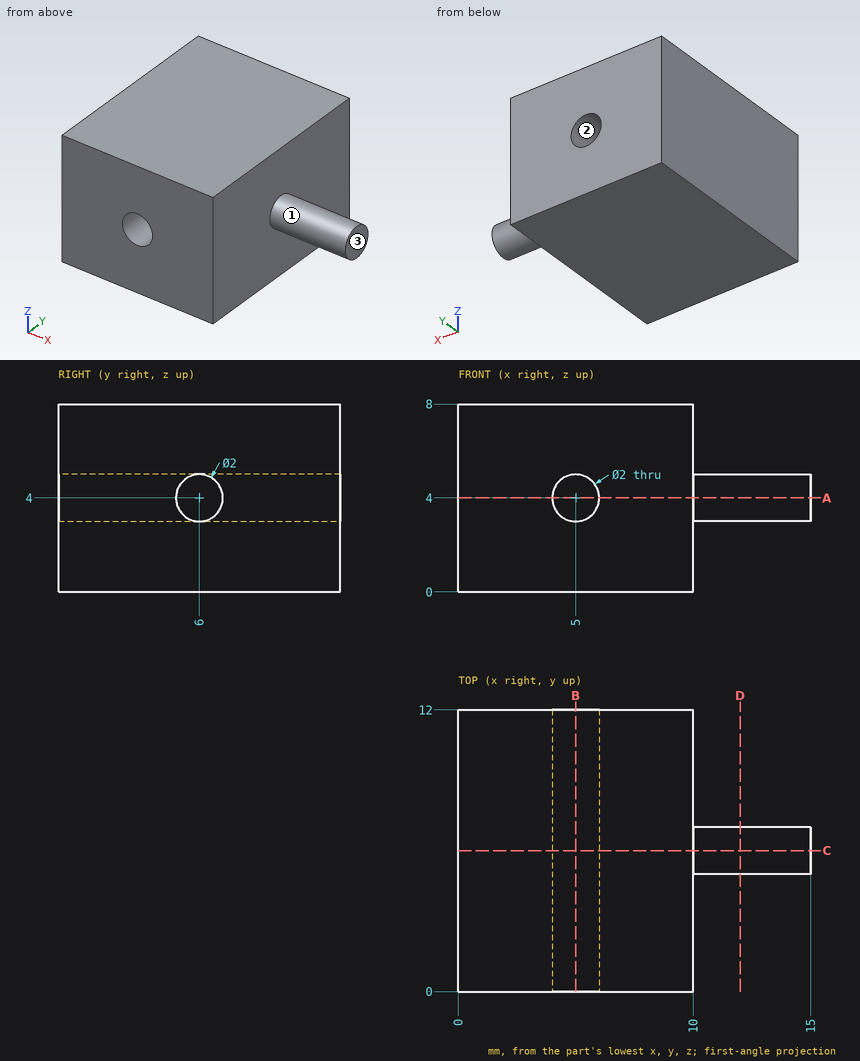
Here's the drawing with two shaded views (mm, measured from the low corner). I have some questions. Coordinates: 2 decimals unless noted, no trailing zeros. Loops run counter-clockwise (first coordinate to the right, second up) from the corner with the lowest first, then second, coordinate; pieces in that order, holes last. Notation, with made-up numbers: (61.25, -37.75) -> (77.25, -37.75) arc R34 ccw to (77.25, -1.75) -> close; hole circle Ø5 at (30.5, 35.5). An arc over 180 degrees is marked (long way). Put each result on its own line as item: value. Start each with the question number.
Q1. I want a section at B-B (x = 5). Write out the boundary of the cut face in (y, z), plus the area to 3 significant figures.
Q2. I'm going to push flat-ended pins straight in: P1, Ø1, axis at y = 7.5, z = 7, coming from the +X side; P2, Ø1.2, axis at x = 5, z = 4, coming from the +Y side. Where does each tip first touch, or does it pass through?
Q3. I want a section at C-C (y = 6). Write out the boundary of the cut face in (x, z).
Q4. I want a section at A-A (z = 4). Write out the boundary of the cut face in (x, y).
Q5. If I drill on line 1 (X direction, y = 4.5, z = 4); line 2 (X direction, y = 6, z = 4); line 3 (X direction, y = 1.75, z = 7), over which ranges is the centre line in solid material (lowest first)? Write a range as [from, to].
Q6. Thinking about a two-plate mould opening in Z: for the marked faces 1, 2 and 3, which applies, pulls with the +Z half, pulls with the -Z half, needs draft (parallel to the pull), parting line crosses it, or undercut?
Q7. I want a section at D-D (x = 12). Write out the boundary of the cut face in (y, z), plus the area to 3 significant figures.
Taken from the geometry:
1. outline: (0, 0) -> (12, 0) -> (12, 3) -> (0, 3) -> close; (0, 5) -> (12, 5) -> (12, 8) -> (0, 8) -> close
1. area: 72.0 mm2
2. P1: stops at x = 10
2. P2: passes through
3. outline: (0, 0) -> (10, 0) -> (10, 3) -> (15, 3) -> (15, 5) -> (10, 5) -> (10, 8) -> (0, 8) -> close; hole circle Ø2 at (5, 4)
4. outline: (0, 0) -> (4, 0) -> (4, 12) -> (0, 12) -> close; (6, 0) -> (10, 0) -> (10, 5) -> (15, 5) -> (15, 7) -> (10, 7) -> (10, 12) -> (6, 12) -> close
5. line 1: x = [0, 4], [6, 10]
5. line 2: x = [0, 4], [6, 15]
5. line 3: x = [0, 10]
6. face 1: parting line crosses it
6. face 2: undercut
6. face 3: needs draft
7. outline: circle Ø2 at (6, 4)
7. area: 3.14 mm2
